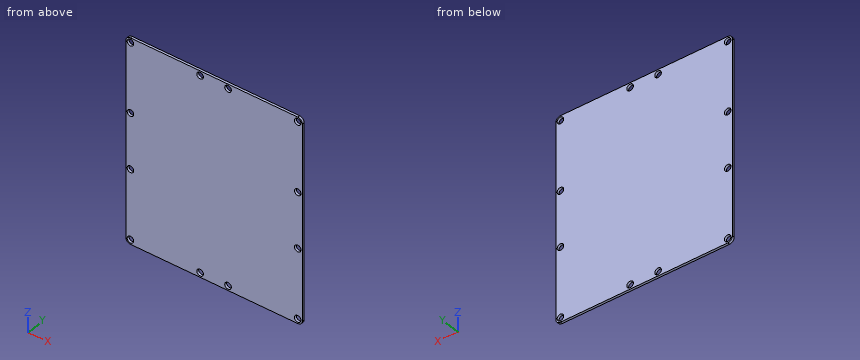
from build123d import *

# Parameters (mm, degrees)
SKETCH1_W             = 120.65
SKETCH1_H             = 139.7
BOSS_EXTRUDE1_DEPTH   = 1.5875
F_8_CLEARANCE_HOLE1_D = 4.4958
FILLET1_R             = 3.175


with BuildPart() as part:
    # Sketch1 → Boss-Extrude1 (new body)
    with BuildSketch(Plane(origin=(0, 0, 0), x_dir=(1, 0, 0), z_dir=(0, 1, 0))):
        Rectangle(SKETCH1_W, SKETCH1_H)
    extrude(amount=BOSS_EXTRUDE1_DEPTH)

    # #8 Clearance Hole1 (through all)
    with Locations(Plane(origin=(0, 1.5875, 0), x_dir=(1, 0, 0), z_dir=(0, 1, 0))):
        with Locations((-57.15, 66.675), (-57.15, 19.05), (-57.15, -19.05), (-57.15, -66.675), (-9.525, -66.675), (9.525, -66.675), (57.15, -66.675), (57.15, -19.05), (57.15, 19.05), (57.15, 66.675), (9.525, 66.675), (-9.525, 66.675)):
            Hole(F_8_CLEARANCE_HOLE1_D / 2)

    # Fillet1
    fillet1_edges = [part.edges().sort_by_distance(p)[0] for p in [
        (-60.325, 0.79375, -69.85),
        (60.325, 0.79375, -69.85),
        (60.325, 0.79375, 69.85),
        (-60.325, 0.79375, 69.85),
    ]]
    fillet(fillet1_edges, radius=FILLET1_R)


solid = part.part
Check sheet for the modelled part. Datum: model origin and axes. Units: mm. Round coordinates to 2 decimals unless told otherwise and drop trailing zeros. Loops run counter-clockwise (first coordinate to the right, second up) from the corner with the lowest first, then second, coordinate; pieces in that order, holes last. Notation, with made-up numbers: M 20,-29 L 49,-29 A35 ccw 49,7 Z; hole C 75.5,77 d6. An arc over 180 degrees is marked long. One line per question, with ' | ' between items. Start each with the question number.
Item 1: Scan lines: probe 1 along X at (y, z) = (0.5, -19.05) (3 decimals); probe 2 along Z at (x, y) = (-57.15, 1); probe 3 along Z at (x, y) = (-8, 1.05). Record each from-to range of solid material in increasing order.
Item 2: Section check A-A (z = -19.05). Record the boundary of the cut face in (x, y) (1 decimal), and give its area (3 significant figures).
Item 3: Section check B-B (x = -9.5). Record the boundary of the cut face in (y, z).
Item 4: Gauge pin test, flat end, axial feed: pin 1 Ø2.5 at (x, z) = (57.15, -19.05) entering from +Y. Record the tip position at first contact, or that the pin passes through.
Worked out:
1) probe 1: -60.325 to -59.398, -54.902 to 54.902, 59.398 to 60.325 | probe 2: -69.85 to -68.92, -64.43 to -21.3, -16.8 to 16.8, 21.3 to 64.43, 68.92 to 69.85 | probe 3: -69.85 to -68.33, -65.02 to 65.02, 68.33 to 69.85
2) outline: M -60.3,0 L -59.4,0 L -59.4,1.6 L -60.3,1.6 Z; M -54.9,0 L 54.9,0 L 54.9,1.6 L -54.9,1.6 Z; M 59.4,0 L 60.3,0 L 60.3,1.6 L 59.4,1.6 Z | area: 177 mm^2
3) outline: M 0,-69.85 L 1.59,-69.85 L 1.59,-68.92 L 0,-68.92 Z; M 0,-64.43 L 1.59,-64.43 L 1.59,64.43 L 0,64.43 Z; M 0,68.92 L 1.59,68.92 L 1.59,69.85 L 0,69.85 Z
4) pin 1: through
